Could you check a few things on this model? Use its own coordinates, in mm. A direction names the side the tool comes from. Give positions to 0.01 mm unless a question says otherwise; leave off trailing zeros. Loops run counter-clockwise (first coordinate to the right, second up) from the corner with the lowest first, then second, coordinate; pieces in that order, holes last. Notation, with made-up numbers: (50.25, -3) - (103.25, -3) arc R25 cw to (103.25, 14) - close; hole circle Ø2 at (79.5, 8.25). An arc over 180 degrees is marked (long way). One line per item, written item: value. Start each with the question number.
Q1. For faces 5 (the face through (23.75, 18, 0)), 6 (the face through (24.736, 30.845, -7.921)), which set-ups out of +Z, -Z, +X, -X, +Y, -Y let a thin tool reach every point of the face, with its end or its side?
Q2. I want a section at A-A (x = 7). Please give me the cut outline in (y, z), then the cut area to 3 significant figures.
Q3. I'm going to push a flat-ended pin straight in: P1, Ø3, axis at x = 0, z = 7, coming from the +Y side. Where does the tip first touch, or does it pass through?
Q4. If we mould it in two halves opening along Y, with no side actions, what happens to faces 1 (the face through (-23.75, 18, 0)), 2 (the face through (24.74, 21.78, -0.27)), 3 (the face through (24.85, 0.86, 0.17)), 4 (the face through (24.74, 35.78, -0.27))? For each: released by +Y, released by -Y, zero draft, split by the parting line, or undercut.
Q5. I want a section at B-B (y = 5). Please give me the cut outline in (x, z), then the cut area to 3 significant figures.
Q6. I want a section at D-D (y = 37). Please give me the cut outline in (x, z).
Q7. I want a section at C-C (z = -7). Please give me the cut outline in (x, y).
Q8. If I drill on line 1 (X direction, y = 18.5, z = 5.5); line 2 (Z direction, x = 0, y = 1.6); line 3 (Y direction, x = -17, z = -3.5), over which ranges is the centre line in solid material (lowest first)? Write a range as from..to.
```python
from build123d import *

# Parameters (mm, degrees)
T_LE_DE_BASE_PLI_E1_DEPTH       = 12
ENL_V_START                     = -51.5
ENL_V_MAT_EXTRU_1_DEPTH         = 51.5
DIAM_TRE_DU_PER_AGE_8_0_8_1_D   = 8
DIAM_TRE_DU_PER_AGE_2_5_2_5_1_D = 2.5
DIAM_TRE_DU_PER_AGE_8_0_8_2_D   = 8
DIAM_TRE_DU_PER_AGE_2_5_2_5_2_D = 2.5


# Read off the part's stored shape, not the designer's step: Enlèv. mat.-Extru.1
# Sheet-metal steps are written as plain solids
with BuildPart() as part:
    # Esquisse1 → Tôle de base pliée1 (new, symmetric)
    with BuildSketch(Plane.XY):
        with BuildLine():
            Line((-25.75, 42), (-25.75, 3))
            ThreePointArc((-25.75, 3), (-24.871320344, 0.878679656), (-22.75, 0))
            Line((-22.75, 0), (22.75, 0))
            ThreePointArc((22.75, 0), (24.871320344, 0.878679656), (25.75, 3))
            Line((25.75, 3), (25.75, 42))
            Line((25.75, 42), (23.75, 42))
            Line((23.75, 42), (23.75, 3))
            ThreePointArc((23.75, 3), (23.457106781, 2.292893219), (22.75, 2))
            Line((22.75, 2), (-22.75, 2))
            ThreePointArc((-22.75, 2), (-23.457106781, 2.292893219), (-23.75, 3))
            Line((-23.75, 3), (-23.75, 42))
            Line((-23.75, 42), (-25.75, 42))
        make_face()
    extrude(amount=T_LE_DE_BASE_PLI_E1_DEPTH, both=True)

    # Enlèv. mat.-Extru.1 outline → Enlèv. mat.-Extru.1 (cut)
    with BuildSketch(Plane(origin=(25.75, 0, 0), x_dir=(0, 0, -1), z_dir=(1, 0, 0)).offset(ENL_V_START)):
        with BuildLine():
            ThreePointArc((-12, 30), (-8.485281374, 38.485281374), (0, 42))
            Line((0, 42), (-12, 42))
            Line((-12, 42), (-12, 30))
        make_face()
        with BuildLine():
            ThreePointArc((0, 42), (8.485281374, 38.485281374), (12, 30))
            Line((12, 30), (12, 42))
            Line((12, 42), (0, 42))
        make_face()
    extrude(amount=ENL_V_MAT_EXTRU_1_DEPTH, mode=Mode.SUBTRACT)

    # Diamètre du perçage Ø8.0 (8)1 (through all)
    with Locations(Plane(origin=(25.75, 0, 0), x_dir=(0, 0, -1), z_dir=(1, 0, 0))):
        with Locations((0, 30)):
            Hole(DIAM_TRE_DU_PER_AGE_8_0_8_1_D / 2)

    # Diamètre du perçage Ø2.5 (2.5)1 (through all)
    with Locations(Plane(origin=(25.75, 0, 0), x_dir=(0, 0, -1), z_dir=(1, 0, 0))):
        with Locations((-7, 30), (0, 37), (7, 30), (0, 23)):
            Hole(DIAM_TRE_DU_PER_AGE_2_5_2_5_1_D / 2)

    # Diamètre du perçage Ø8.0 (8)2 (through all)
    with Locations(Plane(origin=(0, 2, 0), x_dir=(1, 0, 0), z_dir=(0, 1, 0))):
        with Locations((0, 0)):
            Hole(DIAM_TRE_DU_PER_AGE_8_0_8_2_D / 2)

    # Diamètre du perçage Ø2.5 (2.5)2 (through all)
    with Locations(Plane(origin=(0, 2, 0), x_dir=(1, 0, 0), z_dir=(0, 1, 0))):
        with Locations((-7, 0), (0, 7), (7, 0), (0, -7)):
            Hole(DIAM_TRE_DU_PER_AGE_2_5_2_5_2_D / 2)


solid = part.part
```
Worked answers:
1. face 5: +Z, -Z, +Y
1. face 6: +X, -X
2. outline: (0, -12) - (2, -12) - (2, -1.25) - (0, -1.25) - close; (0, 1.25) - (2, 1.25) - (2, 12) - (0, 12) - close
2. area: 43.0 mm²
3. P1: stops at y = 2
4. face 1: zero draft
4. face 2: undercut
4. face 3: released by -Y
4. face 4: undercut
5. outline: (-25.75, -12) - (-23.75, -12) - (-23.75, 12) - (-25.75, 12) - close; (23.75, -12) - (25.75, -12) - (25.75, 12) - (23.75, 12) - close
5. area: 96.0 mm²
6. outline: (-25.75, -9.75) - (-23.75, -9.75) - (-23.75, -1.25) - (-25.75, -1.25) - close; (-25.75, 1.25) - (-23.75, 1.25) - (-23.75, 9.75) - (-25.75, 9.75) - close; (23.75, -9.75) - (25.75, -9.75) - (25.75, -1.25) - (23.75, -1.25) - close; (23.75, 1.25) - (25.75, 1.25) - (25.75, 9.75) - (23.75, 9.75) - close
7. outline: (-25.75, 3) arc R3 ccw to (-22.75, 0) - (-1.25, 0) - (-1.25, 2) - (-22.75, 2) arc R1 cw to (-23.75, 3) - (-23.75, 28.75) - (-25.75, 28.75) - close; (-25.75, 31.25) - (-23.75, 31.25) - (-23.75, 39.75) - (-25.75, 39.75) - close; (1.25, 0) - (22.75, 0) arc R3 ccw to (25.75, 3) - (25.75, 28.75) - (23.75, 28.75) - (23.75, 3) arc R1 cw to (22.75, 2) - (1.25, 2) - close; (23.75, 31.25) - (25.75, 31.25) - (25.75, 39.75) - (23.75, 39.75) - close
8. line 1: x = -25.75..-23.75, 23.75..25.75
8. line 2: z = -12..-8.25, -5.75..-4, 4..5.75, 8.25..12
8. line 3: y = 0..2
